Study the drawing (mm; zero at the part's minimum x, y, z) and answer. Coordinates: 2 decimals unless noted, no trailing zeros. Loops run counter-clockwise (first coordinate to the right, second up) from the corner with the lowest first, then second, coordinate; pieces in that order, holes last. Notation, with made-up numbers: (38.25, 78) - (81.25, 78) arc R24 ccw to (81.25, 117) - close; hole circle Ø5 at (67.25, 77.5). An arc over 180 degrees is marked (long way). Use CSV: the item, a comma, the result in double quotes.
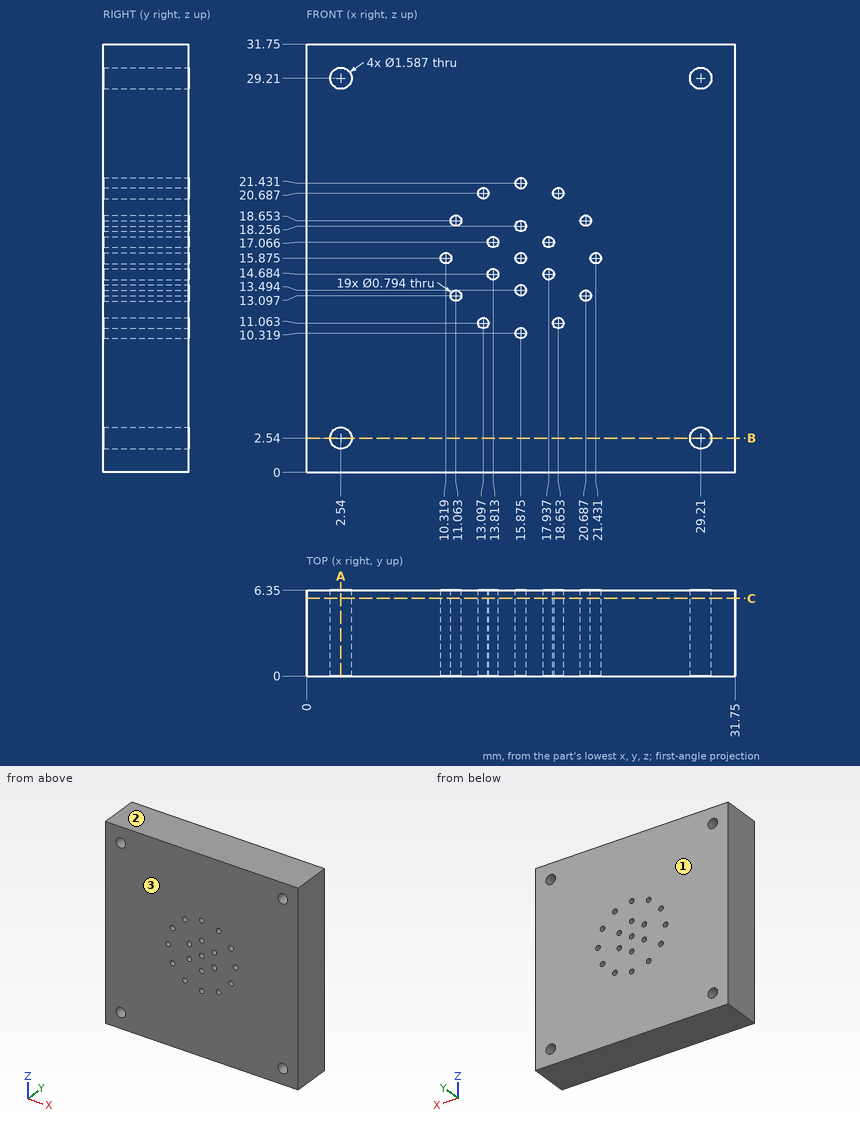
Q1. The part is cut by section A-A on x = 2.54. Determine the outline of the cut face in (y, z).
Reported:
outline,"(0, 0) - (6.35, 0) - (6.35, 1.75) - (0, 1.75) - close; (0, 3.33) - (6.35, 3.33) - (6.35, 28.42) - (0, 28.42) - close; (0, 30) - (6.35, 30) - (6.35, 31.75) - (0, 31.75) - close"
Q2. Given P1, Ø1, axis at x = 29.21, z = 2.54, coming from the -Y side, flat-ended and moving along its own axis, determine where the tip first touches the part or whether it passes through.
Reported:
P1,"passes through"
Q3. For a pull along Y with two mould halves and no side action, classify the marked faces 1, 2 and 3 as +Y half, -Y half, draft (parallel to the pull), parting line (faces both ways), or undercut.
Reported:
face 1,"+Y half"
face 2,"draft"
face 3,"-Y half"
Q4. The part is cut by section C-C on y = 5.75. Give the number of separate pieces and of enclosed holes in the cut face, and give its area (3 significant figures).
Reported:
separate pieces,"1"
enclosed holes,"23"
area,"991 mm²"
Q5. The part is cut by section B-B on z = 2.54. Determine the outline of the cut face in (x, y).
Reported:
outline,"(0, 0) - (1.75, 0) - (1.75, 6.35) - (0, 6.35) - close; (3.33, 0) - (28.42, 0) - (28.42, 6.35) - (3.33, 6.35) - close; (30, 0) - (31.75, 0) - (31.75, 6.35) - (30, 6.35) - close"
Q6. Find the intervals of material crossed by probe 1 along Z at (x, y) = (29.21, 2.5); probe 2 along X at (y, z) = (5.5, 13); probe 3 along X at (y, z) = (1.5, 2), in increasing order. Write a range as [from, to].
Reported:
probe 1,"z = [0, 1.75], [3.33, 28.42], [30, 31.75]"
probe 2,"x = [0, 10.68], [11.45, 20.3], [21.07, 31.75]"
probe 3,"x = [0, 1.96], [3.12, 28.63], [29.79, 31.75]"
